from build123d import *

# Parameters (mm, degrees)
ESQUISSE1_R             = 25.5
BOSS_EXTRU_1_DEPTH      = 2
ESQUISSE2_R             = 15
ESQUISSE2_R_2           = 10
BOSS_EXTRU_2_DEPTH      = 22
ESQUISSE3_R             = 2.5
ENL_V_MAT_EXTRU_1_DEPTH = 2


with BuildPart() as part:
    # Esquisse1 → Boss.-Extru.1 (new body)
    with BuildSketch(Plane.XY):
        Circle(ESQUISSE1_R)
    extrude(amount=BOSS_EXTRU_1_DEPTH)

    # Esquisse2 → Boss.-Extru.2 (add)
    with BuildSketch(Plane(origin=(0, 0, 0), x_dir=(-1, 0, 0), z_dir=(0, 0, -1))):
        Circle(ESQUISSE2_R)
        Circle(ESQUISSE2_R_2, mode=Mode.SUBTRACT)
    extrude(amount=BOSS_EXTRU_2_DEPTH)

    # Esquisse3 → Enlèv. mat.-Extru.1 (cut)
    with BuildSketch(Plane.XY.offset(2)):
        with Locations((0, 18)):
            Circle(ESQUISSE3_R)
    extrude(amount=-ENL_V_MAT_EXTRU_1_DEPTH, mode=Mode.SUBTRACT)


solid = part.part
Source: CAD feature listing. Evaluate the final solid. Frame: model axes, mm. A direction names the side the tool comes from. Round coordinates to 2 decimals unless told otherwise and drop trailing zeros. Order: outer loops, then holes, each group sorted by start corner. A loop starts at its lowest first (then second) coordinate and runs counter-clockwise, first axis right, second up. Notation, with made-up numbers: (72, -34.5) - (106, -34.5) arc R9 ccw to (106, -30.5) - close; hole circle Ø9 at (3, 82). An arc over 180 degrees is marked (long way). Use a Markdown table: item, result. Add a question column.
1. Section query B-B (z = -4). Return the cut outline in (x, y), then the cut area to 3 significant figures.
2. Section query D-D (x = -11). Return the cut outline in (y, z), then the cut area to 3 significant figures.
3. Line query: probe 1 along Y at (x, z) = (0, 0.4); probe 2 along Y at (x, z) = (0, -15.25); probe 3 along Z at (x, y) = (-4, -1). Output: solid intervals per line, ascending.
4. First-contact query: pin 1 (12 mm diameter, centred on y = 9.5, z = -15, fed in from -X); pin 2 (4 mm diameter, centred on y = 9.5, z = -9, fed in from -X); pin 3 (8 mm diameter, centred on x = -4.5, z = -17, fed in from +Y); pin 4 (23 mm diameter, centred on x = 0, y = 0, fed in from -Z). Flat tips, straight axial feed; report the tip coordinate or a pass-through.
5. Mould query, pull axis X, two halves, no side actions, for faces 3 (the cylindrical face through (-0.33, 20.48, 1.01)), 4 (the cylindrical face through (2.17, -9.76, -10.85)), 5 (the cylindrical face through (14.985, 0.66, -10.846)), 6 (the flat face through (0, 0, 2)). Classes: +X half, -X half, draft (parallel to the pull), parting line (faces both ways), or undercut.
6. Section query C-C (y = 0). Return the cut outline in (x, z).
7. Set-up query: faces 1 (the flat face through (-3, -10, -22)), 2 (the flat face through (11, -11, 0)). Return all of +Z, -Z, +X, -X, +Y, -Y with unobstructed straight access to the full face (end or side cutting, diameter ignored); none if empty.
8. Section query A-A (x = 0). Return the cut outline in (y, z).
Derived:
| question | item | result |
|---|---|---|
| 1 | outline | circle Ø30 at (0, 0); hole circle Ø20 at (0, 0) |
| 1 | area | 393 mm2 |
| 2 | outline | (-23.01, 0) - (-10.2, 0) - (-10.2, -22) - (10.2, -22) - (10.2, 0) - (23.01, 0) - (23.01, 2) - (-23.01, 2) - close |
| 2 | area | 541 mm2 |
| 3 | probe 1 | -25.5 to 15.5, 20.5 to 25.5 |
| 3 | probe 2 | -15 to -10, 10 to 15 |
| 3 | probe 3 | 0 to 2 |
| 4 | pin 1 | x = -14.59 |
| 4 | pin 2 | x = -12.99 |
| 4 | pin 3 | y = 14.99 |
| 4 | pin 4 | z = -22 |
| 5 | face 3 | undercut |
| 5 | face 4 | undercut |
| 5 | face 5 | parting line |
| 5 | face 6 | draft |
| 6 | outline | (-25.5, 0) - (-15, 0) - (-15, -22) - (-10, -22) - (-10, 0) - (10, 0) - (10, -22) - (15, -22) - (15, 0) - (25.5, 0) - (25.5, 2) - (-25.5, 2) - close |
| 7 | face 1 | -Z, +X, -X, +Y, -Y |
| 7 | face 2 | -Z |
| 8 | outline | (-25.5, 0) - (-15, 0) - (-15, -22) - (-10, -22) - (-10, 0) - (10, 0) - (10, -22) - (15, -22) - (15, 0) - (15.5, 0) - (15.5, 2) - (-25.5, 2) - close; (20.5, 0) - (25.5, 0) - (25.5, 2) - (20.5, 2) - close |
